from build123d import *

# Parameters (mm, degrees)
SKETCH2_OUTSIDE_W  = 42.182
SKETCH2_OUTSIDE_H  = 42.182
CUT_EXTRUDE1_DEPTH = 44.003953307
SKETCH3_W          = 5
SKETCH3_H          = 6.5


with BuildPart() as part:
    # Sketch1 → Revolve1 (revolve)
    with BuildSketch(Plane(origin=(0, 0, 0), x_dir=(0, 0, -1), z_dir=(1, 0, 0)), mode=Mode.PRIVATE) as revolve1_sk:
        Polygon((-7.5, 10), (-7.3, 10), (-7.3, 14.5), (-0.8, 14.5), (-0.8, 10), (0, 10), (0, 14.5), (30.5, 14.5), (30.5, 6), (-7.5, 6), align=None)
    revolve(revolve1_sk.sketch.rotate(Axis((0, 0, 7.5), (0, 0, -1)), 90), axis=Axis((0, 0, 7.5), (0, 0, -1)))

    # Sketch2 outside → Cut-Extrude1 (cut, through all)
    with BuildSketch(Plane.XY.offset(7.3)):
        Rectangle(SKETCH2_OUTSIDE_W, SKETCH2_OUTSIDE_H)
        Polygon((0, 15.588457268), (-13.5, 7.794228634), (-13.5, -7.794228634), (0, -15.588457268), (13.5, -7.794228634), (13.5, 7.794228634), align=None, mode=Mode.SUBTRACT)
    extrude(amount=-CUT_EXTRUDE1_DEPTH, mode=Mode.SUBTRACT)

    # Sketch3 → Cut-Revolve3 (revolve, cut)
    with BuildSketch(Plane(origin=(0, 0, 0), x_dir=(1, 0, 0), z_dir=(0, 1, 0))):
        with BuildLine():
            Line((-6.75, 30.5), (-6.75, 35.5))
            Line((-6.75, 35.5), (-61.446878064, 35.5))
            Line((-61.446878064, 35.5), (-61.446878064, 23.75))
            Line((-61.446878064, 23.75), (-13.5, 23.75))
            ThreePointArc((-13.5, 23.75), (-11.522970773, 28.522970773), (-6.75, 30.5))
        make_face()
        with Locations((-13.5, 6.5)):
            Rectangle(SKETCH3_W, SKETCH3_H)
    revolve(axis=Axis((0, 0, -30.5), (0, 0, 1)), mode=Mode.SUBTRACT)


solid = part.part
Verification items for the finished model (mm, model axes). A direction names the side the tool comes from. Coordinates: 2 decimals unless noted, no trailing zeros. Order: outer loops, then holes, each group sorted by start corner. A loop starts at its lowest first (then second) coordinate and runs counter-clockwise, first axis right, second up. Notation, with made-up numbers: (68, 47.5) -> (118, 47.5) arc R36 ccw to (118, 83.5) -> close; hole circle Ø11 at (34, 62). An arc over 180 degrees is marked (long way). Use CSV: the item, a comma, the result in double quotes. Start each with the question number.
Q1. Draft check along Z on faces 4 (the flat face through (0, -14, -23.75)), 5 (the cylindrical face through (-9.99, -0.44, 0.39)), 6 (the cylindrical face through (0, 14.5, 4)). Enter one of: +Z half, -Z half, draft (parallel to the pull), parting line (faces both ways), or undercut.
Q2. Tool access check on faces 1 (the flat face through (12, -7, -23.75)), 2 (the cylindrical face through (2.38, 10.74, -6.55)), 3 (the cylindrical face through (12.54, 7.28, -16.85)). Record the directions out of +Z, -Z, +X, -X, +Y, -Y that give a thin tool (end or side, any length) a straight path to the whole face; none if there is none.
Q3. Thickness scan on line 1 along Y through (x, z) = (0, -7.5); line 2 along Y through (x, z) = (0, -20.5); line 3 along Z through (x, y) = (8.75, -7.75). Record the ranges inside material, lowest first.
Q4. Depth check by flat-ended pin: P1, Ø7.5, axis at x = -11, y = -6.5, coming from the -Z side; P2, Ø3, axis at x = -2.5, y = -13.5, coming from the -Z side; P3, Ø3.5, axis at x = 11, y = 5.5, coming from the -Z side; P4, Ø11, axis at x = 0, y = 0, coming from the +Z side. Enter the tip coordinate at first touch or a pass-through.
Q5. Section check A-A, the plane z = 5. Record the cut outline in (x, y).
Returned:
1,face 4,"-Z half"
1,face 5,"undercut"
1,face 6,"draft"
2,face 1,"-Z, +X, -Y"
2,face 2,"none"
2,face 3,"+Z, -Z, +X, +Y"
3,line 1,"y = -11 to -6, 6 to 11"
3,line 2,"y = -14.5 to -6, 6 to 14.5"
3,line 3,"z = -28.35 to -9.75, -3.25 to 0, 0.8 to 7.3"
4,P1,"stops at z = -30.1"
4,P2,"stops at z = -27.69"
4,P3,"stops at z = -29.33"
4,P4,"passes through"
5,outline,"(-13.5, -5.29) arc R14.5 ccw to (-11.33, -9.05) -> (-2.17, -14.34) arc R14.5 ccw to (2.17, -14.34) -> (11.33, -9.05) arc R14.5 ccw to (13.5, -5.29) -> (13.5, 5.29) arc R14.5 ccw to (11.33, 9.05) -> (2.17, 14.34) arc R14.5 ccw to (-2.17, 14.34) -> (-11.33, 9.05) arc R14.5 ccw to (-13.5, 5.29) -> close; hole circle Ø12 at (0, 0)"
